```python
from build123d import *

# Parameters (mm, degrees)
SKETCH_1_R          = 2
SKETCH_1_R_2        = 1
SKETCH_1_W          = 25.5
SKETCH_1_H          = 23
EXTRUDE_1_DEPTH     = 2
SKETCH_3_R          = 1
EXTRUDE_2_DEPTH     = 2.5
SKETCH_4_R          = 2
SKETCH_4_W          = 4
SKETCH_4_H          = 2
EXTRUDE_3_DEPTH     = 3
FILLET_1_R          = 1
FILLET_2_R          = 1
SKETCH_5_W          = 12.5
SKETCH_5_H          = 2.5
EXTRUDE_4_DEPTH     = 2
FILLET_3_R          = 1
SKETCH_6_R          = 2
CUT_EXTRUDE_1_DEPTH = 1
SKETCH_7_R          = 0.75
CUT_EXTRUDE_2_DEPTH = 2.5
SKETCH_8_R          = 0.6
CUT_EXTRUDE_3_DEPTH = 3


with BuildPart() as part:
    # 草图1 → 凸台-拉伸1 (new body)
    with BuildSketch(Plane.XY):
        Polygon((-27, 25), (-15, 25), (-15, 1.5), (-27, 1.5), (-27, -6.5), (-21.5, -12), (-15.5, -12), (-15.5, 0), (15.5, 0), (15.5, -12), (21.5, -12), (27, -6.5), (27, 1.5), (15, 1.5), (15, 25), (27, 25), (27, 28), (22, 33), (-22, 33), (-27, 28), align=None)
        with Locations((20, -7)):
            Circle(SKETCH_1_R, mode=Mode.SUBTRACT)
        with Locations((12.5, 29)):
            Circle(SKETCH_1_R, mode=Mode.SUBTRACT)
        with Locations((0, 29)):
            Circle(SKETCH_1_R, mode=Mode.SUBTRACT)
        with Locations(Location((-20, -7, 0), (0, 0, 180))):
            Circle(SKETCH_1_R, mode=Mode.SUBTRACT)
        with Locations(Location((-12.5, 29, 0), (0, 0, 180))):
            Circle(SKETCH_1_R, mode=Mode.SUBTRACT)
        with Locations((21, 27.5)):
            Circle(SKETCH_1_R_2, mode=Mode.SUBTRACT)
        with Locations((21, -1)):
            Circle(SKETCH_1_R_2, mode=Mode.SUBTRACT)
        with Locations(Location((-21, 27.5, 0), (0, 0, 180))):
            Circle(SKETCH_1_R_2, mode=Mode.SUBTRACT)
        with Locations(Location((-21, -1, 0), (0, 0, 180))):
            Circle(SKETCH_1_R_2, mode=Mode.SUBTRACT)
        with Locations((0, 14)):
            Rectangle(SKETCH_1_W, SKETCH_1_H, mode=Mode.SUBTRACT)
    extrude(amount=EXTRUDE_1_DEPTH)

    # 草图3 → 凸台-拉伸2 (add)
    # profile 1 of 2: a face of its own
    with BuildSketch(Plane(origin=(0, 2.5, 0), x_dir=(1, 0, 0), z_dir=(0, 1, 0))):
        with BuildLine():
            Line((-6.25, -2), (-6.25, -4))
            ThreePointArc((-6.25, -4), (-9.25, -7), (-12.25, -4))
            Line((-12.25, -4), (-12.25, -2))
            Line((-12.25, -2), (-6.25, -2))
        make_face()
        with Locations(Location((-9.25, -4, 0), (0, 0, 180))):
            Circle(SKETCH_3_R, mode=Mode.SUBTRACT)
    # profile 2 of 2: a face of its own
    with BuildSketch(Plane(origin=(0, 2.5, 0), x_dir=(1, 0, 0), z_dir=(0, 1, 0))):
        with BuildLine():
            Line((12.25, -2), (6.25, -2))
            Line((6.25, -2), (6.25, -4))
            ThreePointArc((6.25, -4), (9.25, -7), (12.25, -4))
            Line((12.25, -4), (12.25, -2))
        make_face()
        with Locations((9.25, -4)):
            Circle(SKETCH_3_R, mode=Mode.SUBTRACT)
    extrude(amount=-EXTRUDE_2_DEPTH)

    # 草图4 → 凸台-拉伸3 (add)
    # profile 1 of 3: a face of its own
    with BuildSketch(Plane.XY.offset(2)):
        with BuildLine():
            Line((-15.5, 29), (-15.5, 27))
            Line((-15.5, 27), (-19.480131585, 27))
            ThreePointArc((-19.480131585, 27), (-21, 25.9), (-22.519868415, 27))
            Line((-22.519868415, 27), (-27, 27))
            Line((-27, 27), (-27, 25))
            Line((-27, 25), (-16.5, 25))
            Line((-16.5, 25), (-15, 25))
            Line((-15, 25), (-15, 1.5))
            Line((-15, 1.5), (-27, 1.5))
            Line((-27, 1.5), (-27, -0.5))
            Line((-27, -0.5), (-25, -0.5))
            Line((-25, -0.5), (-22.519868415, -0.5))
            ThreePointArc((-22.519868415, -0.5), (-21, 0.6), (-19.480131585, -0.5))
            Line((-19.480131585, -0.5), (-17.5, -0.5))
            Line((-17.5, -0.5), (-17.5, -4.550510257))
            ThreePointArc((-17.5, -4.550510257), (-21.403955533, -3.793926254), (-23.495572013, -7.176000862))
            Line((-23.495572013, -7.176000862), (-23.495572013, -10.004427987))
            Line((-23.495572013, -10.004427987), (-21.5, -12))
            Line((-21.5, -12), (-15.5, -12))
            Line((-15.5, -12), (-15.5, 0))
            Line((-15.5, 0), (-12.25, 0))
            Line((-12.25, 0), (-12.25, 2.5))
            Line((-12.25, 2.5), (-12.75, 2.5))
            Line((-12.75, 2.5), (-12.75, 25.5))
            Line((-12.75, 25.5), (12.75, 25.5))
            Line((12.75, 25.5), (12.75, 2.5))
            Line((12.75, 2.5), (12.25, 2.5))
            Line((12.25, 2.5), (12.25, 0))
            Line((12.25, 0), (15.5, 0))
            Line((15.5, 0), (15.5, -12))
            Line((15.5, -12), (21.5, -12))
            Line((21.5, -12), (23.495572013, -10.004427987))
            Line((23.495572013, -10.004427987), (23.495572013, -7.176000862))
            ThreePointArc((23.495572013, -7.176000862), (21.403955533, -3.793926254), (17.5, -4.550510257))
            Line((17.5, -4.550510257), (17.5, -0.5))
            Line((17.5, -0.5), (19.480131585, -0.5))
            ThreePointArc((19.480131585, -0.5), (21, 0.6), (22.519868415, -0.5))
            Line((22.519868415, -0.5), (25, -0.5))
            Line((25, -0.5), (27, -0.5))
            Line((27, -0.5), (27, 1.5))
            Line((27, 1.5), (15, 1.5))
            Line((15, 1.5), (15, 25))
            Line((15, 25), (16.5, 25))
            Line((16.5, 25), (27, 25))
            Line((27, 25), (27, 27))
            Line((27, 27), (22.519868415, 27))
            ThreePointArc((22.519868415, 27), (21, 25.9), (19.480131585, 27))
            Line((19.480131585, 27), (15.5, 27))
            Line((15.5, 27), (15.5, 29))
            ThreePointArc((15.5, 29), (11.723542865, 31.897777479), (9.901923789, 27.5))
            Line((9.901923789, 27.5), (2.598076211, 27.5))
            ThreePointArc((2.598076211, 27.5), (0, 32), (-2.598076211, 27.5))
            Line((-2.598076211, 27.5), (-9.901923789, 27.5))
            ThreePointArc((-9.901923789, 27.5), (-11.723542865, 31.897777479), (-15.5, 29))
        make_face()
        with Locations((20, -7)):
            Circle(SKETCH_4_R, mode=Mode.SUBTRACT)
        with Locations((12.5, 29)):
            Circle(SKETCH_4_R, mode=Mode.SUBTRACT)
        with Locations((0, 29)):
            Circle(SKETCH_4_R, mode=Mode.SUBTRACT)
        with Locations(Location((-12.5, 29, 0), (0, 0, 180))):
            Circle(SKETCH_4_R, mode=Mode.SUBTRACT)
        with Locations(Location((-20, -7, 0), (0, 0, 180))):
            Circle(SKETCH_4_R, mode=Mode.SUBTRACT)
    # profile 2 of 3: a face of its own
    with BuildSketch(Plane.XY.offset(2)):
        with Locations((-19, 32)):
            Rectangle(SKETCH_4_W, SKETCH_4_H)
    # profile 3 of 3: a face of its own
    with BuildSketch(Plane.XY.offset(2)):
        with Locations((19, 32)):
            Rectangle(SKETCH_4_W, SKETCH_4_H)
    extrude(amount=EXTRUDE_3_DEPTH)

    # 圆角1
    # the kernel refuses this fillet: 1 mm, written as the material it adds along each edge
    with BuildSketch(Plane(origin=(17.5, -4.550510257, 2), x_dir=(0, 1, 0), z_dir=(0, 0, 1))) as fillet_1_piece_1:
        with BuildLine():
            CenterArc((1.793150944, -1), FILLET_1_R, 90, 109.471220634)
            ThreePointArc((0.850341903, -1.333333333), (0.5014624, -0.618011305), (0, 0))
            Line((0, 0), (1.793150944, 0))
        make_face()
    extrude(amount=3)
    with BuildSketch(Plane(origin=(17.5, -0.5, 2), x_dir=(1, 0, 0), z_dir=(0, 0, 1)), Plane(origin=(15.5, 27, 2), x_dir=(0, 1, 0), z_dir=(0, 0, 1)), Plane(origin=(-15.5, 27, 2), x_dir=(-1, 0, 0), z_dir=(0, 0, 1)), Plane(origin=(-17.5, -0.5, 2), x_dir=(0, -1, 0), z_dir=(0, 0, 1))) as fillet_1_piece_2:
        with BuildLine():
            CenterArc((FILLET_1_R, -FILLET_1_R), FILLET_1_R, 90, 90)
            Line((0, -FILLET_1_R), (0, 0))
            Line((0, 0), (FILLET_1_R, 0))
        make_face()
    extrude(amount=3)
    with BuildSketch(Plane(origin=(9.901923789, 27.5, 2), x_dir=(-1, 0, 0), z_dir=(0, 0, 1)), Plane(origin=(-2.598076211, 27.5, 2), x_dir=(-1, 0, 0), z_dir=(0, 0, 1))) as fillet_1_piece_3:
        with BuildLine():
            CenterArc((1.370550755, -1), FILLET_1_R, 90, 97.180755781)
            ThreePointArc((0.378394014, -1.125), (0.245389674, -0.543599583), (0, 0))
            Line((0, 0), (1.370550755, 0))
        make_face()
    extrude(amount=3)
    with BuildSketch(Plane(origin=(2.598076211, 27.5, 2), x_dir=(0.31880013895525616, 0.9478219618694798, 0), z_dir=(0, 0, 1)), Plane(origin=(-9.901923789, 27.5, 2), x_dir=(0.3188001389552541, 0.9478219618694803, 0), z_dir=(0, 0, 1))) as fillet_1_piece_4:
        with BuildLine():
            CenterArc((1.384753733, -0.980237967), FILLET_1_R, 101.409622109, 97.180755781)
            Line((0.436931771, -1.299038106), (0, 0))
            ThreePointArc((0, 0), (0.593465886, -0.0592861), (1.186931771, 0))
        make_face()
    extrude(amount=3)
    with BuildSketch(Plane(origin=(-17.5, -4.550510257, 2), x_dir=(-0.8431291837491304, 0.5377110557823086, 0), z_dir=(0, 0, 1))) as fillet_1_piece_5:
        with BuildLine():
            CenterArc((1.807326271, -0.974146836), FILLET_1_R, 103.056735384, 109.471220635)
            Line((0.964197087, -1.511857892), (0, 0))
            ThreePointArc((0, 0), (0.790705244, -0.090486073), (1.581410487, 0))
        make_face()
    extrude(amount=3)
    with BuildSketch(Plane(origin=(-21, 33, 2), x_dir=(-1, 0, 0), z_dir=(0, -1, 0)), Plane(origin=(-17, 31, 2), x_dir=(1, 0, 0), z_dir=(0, 1, 0))) as fillet_1_piece_6:
        with BuildLine():
            CenterArc((FILLET_1_R, -FILLET_1_R), FILLET_1_R, 90, 90)
            Line((0, -FILLET_1_R), (0, 0))
            Line((0, 0), (FILLET_1_R, 0))
        make_face()
    extrude(amount=2)
    with BuildSketch(Plane(origin=(17, 31, 2), x_dir=(-1, 0, 0), z_dir=(0, 1, 0)), Plane(origin=(21, 33, 2), x_dir=(1, 0, 0), z_dir=(0, -1, 0))) as fillet_1_piece_7:
        with BuildLine():
            CenterArc((FILLET_1_R, FILLET_1_R), FILLET_1_R, 180, 90)
            Line((0, FILLET_1_R), (0, 0))
            Line((0, 0), (FILLET_1_R, 0))
        make_face()
    extrude(amount=2)
    # the kernel refuses this fillet: 1 mm, written as the material it takes off along each edge
    with BuildSketch(Plane(origin=(-21, 35.5, 5), x_dir=(0, 0, -1), z_dir=(0, -1, 0)), Plane(origin=(21, 35.5, 5), x_dir=(-1, 0, 0), z_dir=(0, -1, 0))) as fillet_1_2_piece_1:
        with BuildLine():
            CenterArc((FILLET_1_R, FILLET_1_R), FILLET_1_R, 180, 90)
            Line((0, FILLET_1_R), (0, 0))
            Line((0, 0), (FILLET_1_R, 0))
        make_face()
    extrude(amount=7, mode=Mode.SUBTRACT)
    with BuildSketch(Plane(origin=(-17, 28.5, 5), x_dir=(-1, 0, 0), z_dir=(0, 1, 0)), Plane(origin=(17, 28.5, 5), x_dir=(0, 0, -1), z_dir=(0, 1, 0))) as fillet_1_2_piece_2:
        with BuildLine():
            CenterArc((FILLET_1_R, -FILLET_1_R), FILLET_1_R, 90, 90)
            Line((0, -FILLET_1_R), (0, 0))
            Line((0, 0), (FILLET_1_R, 0))
        make_face()
    extrude(amount=7, mode=Mode.SUBTRACT)

    # 圆角2
    # the kernel refuses this fillet: 1 mm, written as the material it adds along each edge
    with BuildSketch(Plane(origin=(-12.25, 2.5, 4), x_dir=(0, 0, 1), z_dir=(0, -1, 0))) as fillet_2_piece_1:
        with BuildLine():
            CenterArc((1.830947502, 0.556350833), FILLET_2_R, 213.80380727, 28.955024372)
            ThreePointArc((1.373210626, -0.332736875), (0.706473859, -0.084370619), (0, 0))
            Line((0, 0), (1, 0))
        make_face()
    extrude(amount=2.5)
    with BuildSketch(Plane(origin=(12.25, 2.5, 4), x_dir=(0, 0, 1), z_dir=(0, -1, 0))) as fillet_2_piece_2:
        with BuildLine():
            CenterArc((1.830947502, -0.556350833), FILLET_2_R, 117.241168358, 28.955024372)
            ThreePointArc((1.373210626, 0.332736875), (0.706473859, 0.084370619), (0, 0))
            Line((0, 0), (1, 0))
        make_face()
    extrude(amount=2.5)

    # 草图5 → 凸台-拉伸4 (add)
    with BuildSketch(Plane.XY.offset(2)):
        with Locations((0, 1.25)):
            Rectangle(SKETCH_5_W, SKETCH_5_H)
    extrude(amount=EXTRUDE_4_DEPTH)

    # 圆角3
    fillet_3_edges = [part.edges().sort_by_distance(p)[0] for p in [
        (-6.25, 1.25, 4),
        (6.25, 1.25, 4),
    ]]
    fillet(fillet_3_edges, radius=FILLET_3_R)

    # 草图6 → 切除-拉伸1 (cut)
    with BuildSketch(Plane.XZ):
        with Locations((-9.25, 4)):
            Circle(SKETCH_6_R)
        with Locations((9.25, 4)):
            Circle(SKETCH_6_R)
    extrude(amount=-CUT_EXTRUDE_1_DEPTH, mode=Mode.SUBTRACT)

    # 草图7 → 切除-拉伸2 (cut)
    with BuildSketch(Plane.XZ.offset(12)):
        with Locations((19, 2.5)):
            Circle(SKETCH_7_R)
        with Locations(Location((-19, 2.5, 0), (0, 0, 180))):
            Circle(SKETCH_7_R)
    extrude(amount=-CUT_EXTRUDE_2_DEPTH, mode=Mode.SUBTRACT)

    # 草图8 → 切除-拉伸3 (cut)
    with BuildSketch(Plane(origin=(0, 33, 0), x_dir=(1, 0, 0), z_dir=(0, 1, 0))):
        with Locations(Location((-19, -3, 0), (0, 0, 180))):
            Circle(SKETCH_8_R)
        with Locations(Location((19, -3, 0), (0, 0, 270))):
            Circle(SKETCH_8_R)
    extrude(amount=-CUT_EXTRUDE_3_DEPTH, mode=Mode.SUBTRACT)


solid = part.part
```
Input: part model. Units: mm. Frame: model coordinates. A direction names the side the tool comes from. Coordinates: 2 decimals unless noted, no trailing zeros. Loops run counter-clockwise (first coordinate to the right, second up) from the corner with the lowest first, then second, coordinate; pieces in that order, holes last. Notation, with made-up numbers: M 28.25,89 L 66.25,89 A13 ccw 66.25,106 Z; hole C 12.5,40 d6. An arc over 180 degrees is marked long. One line per item, written item: value.
(1) Pull-direction query (Z, two-part tool) for faces 4 (the cylindrical face through (-8.513, 1.76, 4.676)), 5 (the cylindrical face through (3.21, 27.85, 3.48)), 6 (the flat face through (23, -3, 2)); classes: +Z half, -Z half, draft (parallel to the pull), parting line (faces both ways), or undercut.
Filled in:
face 4: undercut
face 5: draft
face 6: +Z half
(2) Section A-A (z = 1). Give the number of separate pieces and of enclosed holes in the cut face, and give its area (3 significant figures).
Filled in:
separate pieces: 1
enclosed holes: 10
area: 777 mm^2
(3) Line query: line 1 along Y through (x, z) = (-12.5, 1.35); line 2 along Y through (x, z) = (-1, 1.25); line 3 along Z through (x, y) = (-9.25, 1.95). Output: solid intervals per line, ascending. Write a range as from..to.
Filled in:
line 1: 0..2.5, 25.5..27, 31..33
line 2: 0..2.5, 25.5..27.27, 30.73..33
line 3: 0..3, 5..7
(4) Pin query (flat end, axial travel): pin 1 (4.5 mm diameter, centred on x = -12.5, y = 29, fed in from -Z); pin 2 (2.5 mm diameter, centred on x = 21, y = 27.5, fed in from +Z); pin 3 (1.6 mm diameter, centred on x = -19, y = 32, fed in from +Z); pin 4 (0.8 mm diameter, centred on y = 31.5, z = 3.5, fed in from +X). Return the tip coordinate at first contact, or that it passes through.
Filled in:
pin 1: z = 0
pin 2: z = 2
pin 3: z = 5
pin 4: x = 21
(5) Reachability of faces 1 (the cylindrical face through (21, 25.9, 3.5)), 2 (the flat face through (8, 1, 4)), 3 (the flat face through (25, 27, 3)) from +Z, -Z, +X, -X, +Y, -Y: full face, straight path, thin tool, end or side. Return the list, or none.
Filled in:
face 1: +Z
face 2: -Y
face 3: +Z, +X, +Y
(6) Section B-B (y = 11). Output: boundary loops of the cut face in (x, z).
Filled in:
outline: M -15,0 L -12.75,0 L -12.75,5 L -15,5 Z; M 12.75,0 L 15,0 L 15,5 L 12.75,5 Z
(7) Section C-C (x = 0). Output: boundary loops of the cut face in (y, z).
Filled in:
outline: M 0,0 L 2.5,0 L 2.5,4 L 0,4 Z; M 25.5,0 L 27,0 L 27,5 L 25.5,5 Z; M 31,0 L 33,0 L 33,2 L 32,2 L 32,5 L 31,5 Z
